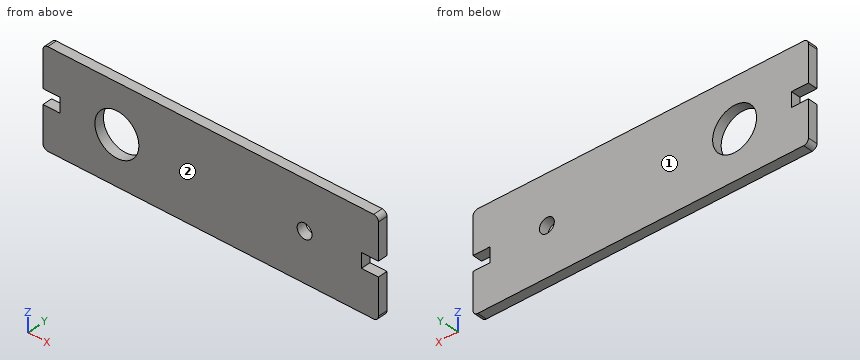
from build123d import *

# Parameters (mm, degrees)
F0_W     = 138.5
F0_H     = 40
F0_R     = 9.075
F0_R_2   = 3.075
F1_DEPTH = 4
F2_R     = 2
F3_W     = 7
F3_H     = 6.05
F4_DEPTH = 25


with BuildPart() as f1:
    # F0 (on Front) → F1 (new body)
    with BuildSketch(Plane.XZ):
        Rectangle(F0_W, F0_H)
        with Locations((-38.75, 0)):
            Circle(F0_R, mode=Mode.SUBTRACT)
        with Locations((38.75, 0)):
            Circle(F0_R_2, mode=Mode.SUBTRACT)
    extrude(amount=F1_DEPTH)

    # F2
    f2_edges = [f1.edges().sort_by_distance(p)[0] for p in [
        (-69.25, -2, -20),
        (-69.25, -2, 20),
        (69.25, -2, -20),
        (69.25, -2, 20),
    ]]
    fillet(f2_edges, radius=F2_R)

    # F3 (on face) → F4 (cut)
    with BuildSketch(Plane.XZ.offset(4)):
        with Locations((-65.75, 0)):
            Rectangle(F3_W, F3_H)
        with Locations((65.75, 0)):
            Rectangle(F3_W, F3_H)
    extrude(amount=-F4_DEPTH, mode=Mode.SUBTRACT)


solid = f1.part
Geometry: final body of the model. Coordinates: model frame, mm. Face numbers are marked on the shaded views. Round coordinates to 2 decimals unless told otherwise and drop trailing zeros. Write each loop counter-clockwise with the first axis right and the second up, starting at its lowest first coordinate (ties: lowest second). Pieces come first, ordered by that corner, then holes. Notation, with made-up numbers: M -14,8.25 L -5,8.25 A4 cw -5,14.25 Z; hole C -17.5,35.25 d1. An arc over 180 degrees is marked long. Write item = value, one per line.
Item 1: Pin query (flat end, axial travel): P1, Ø1.2, axis at y = -2.5, z = 1.5, coming from the +X side; P2, Ø16.5, axis at x = -38.75, z = 0, coming from the -Y side. Return the tip coordinate at first contact, or that it passes through.
Findings:
P1 = 62.25
P2 = through
Item 2: Section query D-D on z = -7. Return loops of the section in (x, y), then the cut area to 3 significant figures.
Findings:
outline = M -69.25,-4 L -44.53,-4 L -44.53,0 L -69.25,0 Z; M -32.97,-4 L 69.25,-4 L 69.25,0 L -32.97,0 Z
area = 508 mm^2
Item 3: Section query C-C on y = -1.2. Return loops of the section in (x, z) (3 decimals).
Findings:
outline = M -69.25,-18 A2 ccw -67.25,-20 L 67.25,-20 A2 ccw 69.25,-18 L 69.25,-3.025 L 62.25,-3.025 L 62.25,3.025 L 69.25,3.025 L 69.25,18 A2 ccw 67.25,20 L -67.25,20 A2 ccw -69.25,18 L -69.25,3.025 L -62.25,3.025 L -62.25,-3.025 L -69.25,-3.025 Z; hole C -38.75,0 d18.15; hole C 38.75,0 d6.15
Item 4: Section query A-A on x = -38.75. Return loops of the section in (y, z) (3 decimals), then the cut area to 3 significant figures.
Findings:
outline = M -4,-20 L 0,-20 L 0,-9.075 L -4,-9.075 Z; M -4,9.075 L 0,9.075 L 0,20 L -4,20 Z
area = 87.4 mm^2
Item 5: Section query B-B on z = 0. Return loops of the section in (x, y) (3 decimals).
Findings:
outline = M -62.25,-4 L -47.825,-4 L -47.825,0 L -62.25,0 Z; M -29.675,-4 L 35.675,-4 L 35.675,0 L -29.675,0 Z; M 41.825,-4 L 62.25,-4 L 62.25,0 L 41.825,0 Z
Item 6: Pull-direction query (Y, two-part tool) for the marked faces 1 and 2; classes: pulls with the +Y half, pulls with the -Y half, needs draft (parallel to the pull), parting line crosses it, or undercut.
Findings:
face_1 = pulls with the +Y half
face_2 = pulls with the -Y half
Item 7: Material intervals for line 1 along Z through (x, y) = (38.75, -2.15) (3 decimals); line 2 along Z through (x, y) = (-38.75, -1.8) (3 decimals); line 3 along X through (y, z) = (-2.1, 1), sorted ascending. Write a range as [from, to].
Findings:
line_1 = [-20, -3.075], [3.075, 20]
line_2 = [-20, -9.075], [9.075, 20]
line_3 = [-62.25, -47.77], [-29.73, 35.84], [41.66, 62.25]
